The listing builds one solid part. Answer for the finished solid, in the listing's coordinates (mm). A direction names the side the tool comes from. Round coordinates to 2 decimals unless told otherwise and drop trailing zeros. Order: outer loops, then holes, each group sorted by start corner. A loop starts at its lowest first (then second) coordinate and runs counter-clockwise, first axis right, second up. Notation, with made-up numbers: M 51.5,11 L 60.5,11 A12 cw 60.5,31 Z; hole C 67.25,28.25 d6. An arc over 180 degrees is marked long. Write item = value, one per line. Start each with the question number.
(1) This flat-tipped pin is pushed along its axis until it touches: pin 1 (1.2 mm diameter, centred on x = 2, y = 1.5, fed in from +Z). Where does it stop, or does it pass through?
(2) A cutting plane is placed at C-C, the plane x = 2. Count the separate pieces of the cut face and the enclosed holes in it, and give its area (3 significant figures).
(3) A cutting plane is placed at A-A, the plane y = 3.5. Determine the outline of the cut face in (x, z).
(4) For a pull along Y with two mould halves and no side action, classify faces 1 (the face through (2, 7.4, 3.5)), 2 (the face through (2, 6, 3.5)), 3 (the face through (2, 11, 1)), 4 (the face through (2, 2.5, 3)) as released by +Y, released by -Y, zero draft, split by the parting line, or undercut.
(5) Straight lines are drawn through the part: probe 1 along X at (y, z) = (3.5, 1.15); probe 2 along Y at (x, z) = (1.8, 0.2); probe 3 along Y at (x, z) = (2, 1.5) (3 decimals). For each, find the intervals that lie inside material, in ascending order. Write a range as from..to.
(6) A cutting plane is placed at B-B, the plane z = 1.7. Determine the outline of the cut face in (x, y) (3 decimals).
(7) Which of the six approach directions +Z, -Z, +X, -X, +Y, -Y give full straight-line access (tool end or side, diameter ignored) to faces 5 (the face through (1.5, 6.7, 3)), 6 (the face through (2, 6, 0)), 7 (the face through (1.5, 9.7, 3))?
(8) A cutting plane is placed at D-D, the plane x = 0.3. Determine the outline of the cut face in (y, z), and give its area (4 significant figures).
Autodesk Inventor part; units mm, degrees
ref_plane "YZ Plane" through (0, 0, 0) normal (1, 0, 0) x (0, 1, 0)
ref_plane "XZ Plane" through (0, 0, 0) normal (0, 1, 0) x (-1, 0, 0)
ref_plane "XY Plane" through (0, 0, 0) normal (0, 0, 1) x (1, 0, 0)
sketch "스케치1" plane through (0, 0, 0) normal (0, 0, 1) x (1, 0, 0)
  line L0 (0, 0) -> (4, 0)
  line L1 (4, 0) -> (4, 11)
  line L2 (4, 11) -> (0, 11)
  line L3 (0, 11) -> (0, 0)
  dimension "d0" = 4
  dimension "d1" = 11
extrude "돌출1" add sketch "스케치1" along normal blind 3
sketch "스케치2" plane through (0, 0, 3) normal (0, 0, 1) x (1, 0, 0)
  line L0 (4, 11) -> (0, 11) construction
  line L1 (2, 11) -> (2, 0) construction
  line L2 (0, 0) -> (4, 0) construction
  line L3 (0, 6) -> (4, 6)
  line L4 (4, 6) -> (4, 5)
  line L5 (4, 5) -> (0, 5)
  line L6 (0, 5) -> (0, 6)
  line L7 (4, 0) -> (4, 11)
  line L8 (0, 11) -> (0, 0)
  point P0 (2, 6.7)
  point P1 (2, 3.5)
  point P2 (2, 1.3)
  point P3 (2, 6.7)
  point P4 (2, 9.7)
  dimension "d7" = 1
  dimension "d8" = 5
  dimension "d9" = 4.3
  dimension "d45" = 1.3
  dimension "d51" = 3.2
  dimension "d52" = 2.2
  dimension "d54" = 0
  dimension "d55" = 1.3
extrude "돌출2" add sketch "스케치2" along normal blind 1
hole "구멍1" at (2, 6.7, 3) direction (0, 0, -1) diameter 0.63 end through all
hole "구멍2" at (2, 3.5, 3) direction (0, 0, -1) diameter 1.6 end through all
hole "구멍3" at (2, 1.3, 3) at (2, 9.7, 3) direction (0, 0, -1) diameter 0.65 end through all
chamfer "모따기1" distance 0.5 angle 45 1 edges at (2, 5, 4)
ref_plane "작업 평면1" through (0, 6.7, 3) normal (0, 1, 0) x (1, 0, 0)
mirror "미러1" about plane through (0, 6.7, 3) normal (0, 1, 0) of "돌출2", "모따기1"
equation "\"G23_M\" = 0.67"
equation "\"G23_F\" = 0.65"
properties part number "_3D 인쇄"
Reported:
q1.pin_1 = 3
q2.separate_pieces = 5
q2.enclosed_holes = 0
q2.area = 24.2 mm²
q3.outline = M 0,0 L 1.2,0 L 1.2,3 L 0,3 Z; M 2.8,0 L 4,0 L 4,3 L 2.8,3 Z
q4.face_1 = undercut
q4.face_2 = undercut
q4.face_3 = released by +Y
q4.face_4 = zero draft
q5.probe_1 = 0..1.2, 2.8..4
q5.probe_2 = 0..1.04, 1.56..2.73, 4.27..6.46, 6.94..9.44, 9.96..11
q5.probe_3 = 0..0.975, 1.625..2.7, 4.3..6.385, 7.015..9.375, 10.025..11
q6.outline = M 0,0 L 4,0 L 4,11 L 0,11 Z; hole C 2,3.5 d1.6; hole C 2,1.3 d0.65; hole C 2,9.7 d0.65; hole C 2,6.7 d0.63
q7.face_5 = +Z, +X, -X
q7.face_6 = -Z, +X, -X, +Y, -Y
q7.face_7 = +Z, +X, -X, +Y
q8.outline = M 0,0 L 11,0 L 11,3 L 8.4,3 L 8.4,3.5 L 7.9,4 L 7.4,4 L 7.4,3 L 6,3 L 6,4 L 5.5,4 L 5,3.5 L 5,3 L 0,3 Z
q8.area = 34.75 mm²
